Verification items for the finished model (mm, model axes). A direction names the side the tool comes from. Coordinates: 2 decimals unless noted, no trailing zeros. Order: outer loops, then holes, each group sorted by start corner. A loop starts at its lowest first (then second) coordinate and runs counter-clockwise, first axis right, second up. Notation, with made-up numbers: (54.5, 47) -> (64.5, 47) arc R8 cw to (64.5, 52) -> close; hole circle Ø5 at (16.5, 28). An arc over 180 degrees is marked (long way). Use CSV: the item, a comma, the result in double quotes. Start each with the question number.
1) Scan lines: line 1 along Z through (x, y) = (-13.95, 20.75); line 2 along Y through (x, z) = (-11.5, -1.5); line 3 along X through (y, z) = (20.15, 0). Record each from-to range of solid material in increasing order.
2) Sectioned sample at B-B on y = 10.5. Record the boundary of the cut face in (x, z), then the cut area to 3 significant figures.
3) Sectioned sample at A-A on x = -13.95. Record the boundary of the cut face in (y, z), then the cut area to 3 significant figures.
4) Sectioned sample at D-D on x = -0.7. Record the boundary of the cut face in (y, z), then the cut area to 3 significant figures.
5) Go/stop test with flat-tipped pins: pin 1 (5 mm diameter, centred on y = 10.5, z = 1, fed in from -X); pin 2 (3 mm diameter, centred on x = -0.5, z = -3, fed in from +Y); pin 3 (3 mm diameter, centred on x = 10, z = 2, fed in from +Y). Record where each tip stops, or that it passes through.
6) Sectioned sample at C-C on z = -2. Record the boundary of the cut face in (x, y).
7) Tool access check on faces 1 (the flat face through (-11.6, 10, 0)), 2 (the flat face through (1.6, 27.7, -3.2)), 3 (the flat face through (15.4, 20.5, -0.7)), 4 (the flat face through (11.6, 10, 0)). Record the directions out of +Z, -Z, +X, -X, +Y, -Y that give a thin tool (end or side, any length) a straight path to the whole face; none if there is none.
Autodesk Inventor part; units mm, degrees
ref_plane "YZ Plane" through (0, 0, 0) normal (1, 0, 0) x (0, 1, 0)
ref_plane "XZ Plane" through (0, 0, 0) normal (0, 1, 0) x (-1, 0, 0)
ref_plane "XY Plane" through (0, 0, 0) normal (0, 0, 1) x (1, 0, 0)
sketch "Sketch1" plane through (0, 0, 0) normal (0, 1, 0) x (-1, 0, 0)
  line L0 (-11.6, -6.2) -> (11.6, -6.2)
  line L1 (11.6, -6.2) -> (11.6, 6.2)
  line L2 (11.6, 6.2) -> (-11.6, 6.2)
  line L3 (-11.6, 6.2) -> (-11.6, -6.2)
  line L4 (-11.6, -6.2) -> (11.6, 6.2) construction
  line L5 (11.6, -6.2) -> (-11.6, 6.2) construction
  point P0 (0, 0)
extrude "Extrusion1" add sketch "Sketch1" along normal blind 31.7
sketch "Sketch2" plane through (11.6, 0, 6.2) normal (1, 0, 0) x (0, 0, -1)
  line L0 (12.4, 19.4) -> (0, 19.4)
  line L1 (0, 19.4) -> (0, 21.5)
  line L2 (0, 21.5) -> (12.4, 21.5)
  line L3 (12.4, 21.5) -> (12.4, 19.4)
extrude "Extrusion2" add sketch "Sketch2" along normal blind 4.4
sketch "Sketch8" plane through (-11.6, 0, -6.2) normal (-1, 0, 0) x (0, 0, 1)
  line L0 (12.4, 19.4) -> (0, 19.4)
  line L1 (0, 19.4) -> (0, 21.5)
  line L2 (0, 21.5) -> (12.4, 21.5)
  line L3 (12.4, 21.5) -> (12.4, 19.4)
  point P0 (12.4, 0)
  point P1 (6.2, 0)
extrude "Extrusion3" add sketch "Sketch8" along normal blind 4.4
sketch "Sketch10" plane through (0, 31.7, 0) normal (0, 1, 0) x (1, 0, 0)
  circle A0 centre (5.4, 0) radius 6.2
sketch "Sketch11" plane through (0, 31.7, 0) normal (0, 1, 0) x (1, 0, 0)
  circle A0 centre (-0.7, 0) radius 3.1
  point P0 (0, 0)
sketch "Sketch12" plane through (0, 31.7, 0) normal (0, 1, 0) x (1, 0, 0)
  line L0 (11.6, 6.2) -> (-11.6, 6.2)
  line L1 (-11.6, 6.2) -> (-11.6, -6.2)
  line L2 (-11.6, -6.2) -> (11.6, -6.2)
  line L3 (11.6, -6.2) -> (11.6, 6.2)
  point P0 (0, 0)
extrude "Extrusion4" cut sketch "Sketch12" against normal blind 7.9
extrude "Extrusion5" add sketch "Sketch10" against normal blind 7.9
extrude "Extrusion6" add sketch "Sketch11" against normal blind 7.9
sketch "Sketch13" plane through (0, 31.7, 0) normal (0, 1, 0) x (1, 0, 0)
  arc A0 (-0.0131, -3.0229) -> (-0.0131, 3.0229) centre (5.4, 0) ccw
  arc A1 (-0.0131, 3.0229) -> (-0.0131, -3.0229) centre (-0.7, 0) ccw
  circle A2 centre (5.4, 0) radius 4.75
  circle A3 centre (-0.7, 0) radius 1.35
extrude "Extrusion7" cut sketch "Sketch13" against normal blind 4
sketch "Sketch14" plane through (5.4, 31.7, 0) normal (0, 1, 0) x (1, 0, 0)
  circle A0 centre (0, 0) radius 4.75
  circle A1 centre (0, 0) radius 2.5
  point P0 (-4.75, 0)
  point P1 (-5.4, 0)
  dimension "d28" = 5
extrude "Extrusion8" cut sketch "Sketch14" against normal blind 3
sketch "Sketch15" plane through (-0.7, 31.7, 0) normal (0, 1, 0) x (1, 0, 0)
  circle A0 centre (0, 0) radius 1.35
extrude "Extrusion9" cut sketch "Sketch15" against normal blind 3
sketch "Sketch16" plane through (11.6, 21.5, 6.2) normal (0, 1, 0) x (1, 0, 0)
  circle A0 centre (2.35, 6.2) radius 1.15
  line L0 (4.4, 6.2) -> (4.4, 5.5)
  line L1 (4.4, 5.5) -> (3.2624, 5.5)
  line L2 (4.4, 6.2) -> (4.4, 6.9)
  line L3 (4.4, 6.9) -> (3.2624, 6.9)
  point P0 (-11.6, 6.2)
sketch "Sketch17" plane through (-11.6, 21.5, 6.2) normal (0, 1, 0) x (1, 0, 0)
  circle A0 centre (-2.35, 6.2) radius 1.15
  line L0 (-4.4, 6.2) -> (-4.4, 6.9)
  line L1 (-4.4, 6.9) -> (-3.2624, 6.9)
  line L2 (-4.4, 6.2) -> (-4.4, 5.5)
  line L3 (-4.4, 5.5) -> (-3.2624, 5.5)
  point P0 (11.6, 6.2)
sketch "Sketch18" plane through (-11.6, 21.5, 6.2) normal (0, 1, 0) x (1, 0, 0)
  point P0 (11.6, 6.2)
extrude "Extrusion10" cut sketch "Sketch17" against normal blind 3
extrude "Extrusion11" cut sketch "Sketch16" against normal blind 3
fillet "Fillet1" radius 1 1 edges at (-16, 20.45, -6.2)
sketch "Sketch20" plane through (-11.6, 21.5, 6.2) normal (0, 1, 0) x (1, 0, 0)
  point P0 (11.6, 6.2)
fillet "Fillet2" radius 1 1 edges at (16, 20.45, -6.2)
fillet "Fillet3" radius 1 1 edges at (-16, 20.45, 6.2)
fillet "Fillet4" radius 1 1 edges at (16, 20.45, 6.2)
fillet "Fillet5" radius 1 1 edges at (11.6, 22.65, 6.2)
fillet "Fillet6" radius 1 1 edges at (11.6, 22.65, -6.2)
fillet "Fillet7" radius 1 1 edges at (-11.6, 22.65, 6.2)
fillet "Fillet8" radius 1 1 edges at (-11.6, 22.65, -6.2)
fillet "Fillet9" radius 1 1 edges at (-11.6, 9.7, -6.2)
fillet "Fillet10" radius 1 1 edges at (11.6, 9.7, -6.2)
fillet "Fillet11" radius 1 1 edges at (11.6, 9.7, 6.2)
fillet "Fillet12" radius 1 1 edges at (-11.6, 9.7, 6.2)
properties part number "micro_servo"
Answers follow:
1,line 1,"z = -6.2 to -1.15, 1.15 to 6.2"
1,line 2,"y = 0 to 23.8"
1,line 3,"x = -12.8 to 12.8"
2,outline,"(-11.6, -5.2) arc R1 ccw to (-10.6, -6.2) -> (10.6, -6.2) arc R1 ccw to (11.6, -5.2) -> (11.6, 5.2) arc R1 ccw to (10.6, 6.2) -> (-10.6, 6.2) arc R1 ccw to (-11.6, 5.2) -> close"
2,area,"287 mm²"
3,outline,"(19.4, -6.2) -> (21.5, -6.2) -> (21.5, -1.15) -> (19.4, -1.15) -> close; (19.4, 1.15) -> (21.5, 1.15) -> (21.5, 6.2) -> (19.4, 6.2) -> close"
3,area,"21.2 mm²"
4,outline,"(0, -6.2) -> (23.8, -6.2) -> (23.8, -3.1) -> (27.7, -3.1) -> (27.7, -1.35) -> (28.7, -1.35) -> (28.7, 1.35) -> (27.7, 1.35) -> (27.7, 3.1) -> (23.8, 3.1) -> (23.8, 6.2) -> (0, 6.2) -> close"
4,area,"322 mm²"
5,pin 1,"stops at x = -11.6"
5,pin 2,"stops at y = 27.7"
5,pin 3,"stops at y = 28.7"
6,outline,"(-16, 19.4) -> (-11.6, 19.4) -> (-11.6, 0) -> (11.6, 0) -> (11.6, 19.4) -> (16, 19.4) -> (16, 21.5) -> (11.6, 21.5) -> (11.6, 23.8) -> (11.27, 23.8) -> (11.27, 27.7) -> (9.71, 27.7) -> (9.71, 28.7) -> (6.9, 28.7) -> (6.9, 31.7) -> (3.9, 31.7) -> (3.9, 28.7) -> (1.09, 28.7) -> (1.09, 27.7) -> (-3.07, 27.7) -> (-3.07, 23.8) -> (-11.6, 23.8) -> (-11.6, 21.5) -> (-16, 21.5) -> close"
7,face 1,"+Z, -Z, -X, -Y"
7,face 2,"+Y"
7,face 3,"+X, +Y, -Y"
7,face 4,"+Z, -Z, +X, -Y"
